Answer from the drawing. Dimensions are ordinates in mm from the lowest x, y and z of the part. Coordinates: 2 decimals unless noted, no trailing zeros. Order: outer loops, then holes, each group sorted by start corner. A loop starts at its lowest first (then second) coordinate and runs counter-clockwise, first axis right, second up. Notation, with made-up numbers: (59.5, -15.75) - (113.5, -15.75) arc R17 ccw to (113.5, 2.25) - close; hole circle Ø6 at (-4, 80). An arc over 180 degrees is marked (long way). Use a Markdown table: item, result. Add a question column.
Item 1: The part is cut by section D-D, the plane y = 33.5. Give the vertices of the cut face in (x, z).
Item 2: Find the intervals of material crossed by line 1 along Y through (x, z) = (153.5, 4.1); line 2 along X through (y, z) = (92, 2.1); line 3 along X through (y, z) = (95, 1.7), in increasing order.
Item 3: The part is cut by section A-A, the plane z = 2.95. State how many separate pieces and enclosed holes the cut face has, then the cut area to 3 significant figures.
Item 4: The part is cut by section C-C, the plane x = 41. Give the vertices of the cut face in (y, z), then the cut area to 3 significant figures.
Item 5: Flat-ended cylindrical pins translate along their axes: P1, Ø3.5, axis at x = 171.25, y = 92, coming from the +Z side; P2, Ø4, axis at x = 143.5, y = 84.5, coming from the +Z side. Find the tip coordinate at first contact, or state that the pin passes through.
Item 6: The part is cut by section B-B, the plane y = 64.5. Give the vertices of the cut face in (x, z).
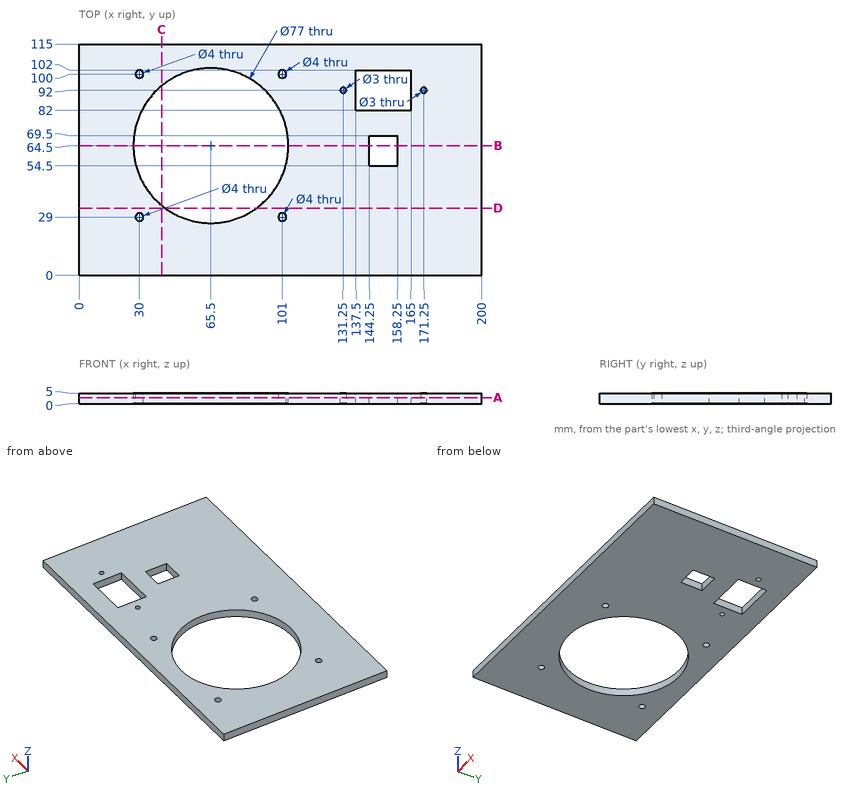
Solution:
| question | item | result |
|---|---|---|
| 1 | outline | (0, 0) - (42.67, 0) - (42.67, 5) - (0, 5) - close; (88.33, 0) - (200, 0) - (200, 5) - (88.33, 5) - close |
| 2 | line 1 | y = 0 to 54.5, 69.5 to 82, 102 to 115 |
| 2 | line 2 | x = 0 to 38.56, 92.44 to 129.75, 132.75 to 137.5, 165 to 169.75, 172.75 to 200 |
| 2 | line 3 | x = 0 to 42.01, 88.99 to 137.5, 165 to 200 |
| 3 | separate pieces | 1 |
| 3 | enclosed holes | 9 |
| 3 | area | 17,500 mm2 |
| 4 | outline | (0, 0) - (34.8, 0) - (34.8, 5) - (0, 5) - close; (94.2, 0) - (115, 0) - (115, 5) - (94.2, 5) - close |
| 4 | area | 278 mm2 |
| 5 | P1 | stops at z = 5 |
| 5 | P2 | passes through |
| 6 | outline | (0, 0) - (27, 0) - (27, 5) - (0, 5) - close; (104, 0) - (144.25, 0) - (144.25, 5) - (104, 5) - close; (158.25, 0) - (200, 0) - (200, 5) - (158.25, 5) - close |
